Can you work these out from the model? Positions are in its coordinate system, mm. Face numbers are marked on the shaded views. A direction names the side the tool comes from. Coordinates: 2 decimals unless noted, no trailing zeros. Write each loop counter-clockwise with the first axis right and the second up, starting at its lowest first coordinate (ties: lowest second). Pieces come first, ordered by that corner, then holes. Notation, with made-up numbers: (-17, 86) -> (29, 86) arc R23 ccw to (29, 115) -> close; hole circle Ø11 at (73.25, -13.5). An arc over 180 degrees is marked (long way). Use one line per item in the form item = value.
```python
from build123d import *

# Parameters (mm, degrees)
SKETCH1_R           = 12
BOSS_EXTRUDE1_DEPTH = 5
BOSS_EXTRUDE2_DEPTH = 2
BOSS_EXTRUDE3_DEPTH = 2
SKETCH4_R           = 15.547757557
SKETCH4_R_2         = 12
BOSS_EXTRUDE4_DEPTH = 10
SKETCH5_W           = 10
SKETCH5_H           = 9.018962752
BOSS_EXTRUDE5_DEPTH = 2
SKETCH6_W           = 25.14370714
SKETCH6_H           = 10
BOSS_EXTRUDE6_DEPTH = 2
CUT_EXTRUDE1_DEPTH  = 2
CUT_EXTRUDE2_DEPTH  = 0.2


with BuildPart() as part:
    # Sketch1 → Boss-Extrude1 (new body)
    with BuildSketch(Plane.XY):
        with BuildLine():
            Line((-27.15, 21.666502105), (-25.112032094, 30.452193651))
            ThreePointArc((-25.112032094, 30.452193651), (-11.263369735, 42.043284959), (3.691801624, 31.919960581))
            Line((3.691801624, 31.919960581), (27.293258902, 23.278095711))
            Line((27.293258902, 23.278095711), (27.293258902, 10))
            Line((27.293258902, 10), (27.293258902, -9.955183239))
            Line((27.293258902, -9.955183239), (20.497693749, -9.955183239))
            Line((20.497693749, -9.955183239), (20.497693749, 10))
            Line((20.497693749, 10), (-20.5, 10))
            Line((-20.5, 10), (-20.5, -9.955183239))
            Line((-20.5, -9.955183239), (-27.15, -9.955183239))
            Line((-27.15, -9.955183239), (-27.15, 10))
            Line((-27.15, 10), (-27.15, 21.666502105))
        make_face()
        with Locations((-10.5, 27.062721997)):
            Circle(SKETCH1_R, mode=Mode.SUBTRACT)
    extrude(amount=BOSS_EXTRUDE1_DEPTH)

    # Sketch2 → Boss-Extrude2 (add)
    with BuildSketch(Plane(origin=(27.293258902, 0, 0), x_dir=(0, 0, -1), z_dir=(1, 0, 0))):
        Polygon((-5, -9.955183239), (-5, 23.278095711), (-15, 23.278095711), align=None)
    extrude(amount=-BOSS_EXTRUDE2_DEPTH)

    # Sketch3 → Boss-Extrude3 (add)
    with BuildSketch(Plane.ZY.offset(27.15)):
        Polygon((5, -9.955183239), (5, 23.278095711), (15, 23.278095711), align=None)
    extrude(amount=-BOSS_EXTRUDE3_DEPTH)

    # Sketch4 → Boss-Extrude4 (add)
    with BuildSketch(Plane.XY.offset(5)):
        with Locations((-10.5, 27.062721997)):
            Circle(SKETCH4_R)
        with Locations((-10.5, 27.062721997)):
            Circle(SKETCH4_R_2, mode=Mode.SUBTRACT)
    extrude(amount=BOSS_EXTRUDE4_DEPTH)

    # Sketch5 → Boss-Extrude5 (add)
    with BuildSketch(Plane(origin=(-30.532955865, 7.082559615, 0), x_dir=(0, 0, 1), z_dir=(-0.9741354729183627, 0.22596477690586622, 0))):
        with Locations((10, 21.050556457)):
            Rectangle(SKETCH5_W, SKETCH5_H)
    extrude(amount=-BOSS_EXTRUDE5_DEPTH)

    # Sketch6 → Boss-Extrude6 (add)
    with BuildSketch(Plane(origin=(10.742458336, 29.338305481, 0), x_dir=(0.9390305732894374, -0.34383365517021547, 0), z_dir=(0.34383365517021547, 0.9390305732894374, 0))):
        with Locations((5.053558251, -10)):
            Rectangle(SKETCH6_W, SKETCH6_H)
    extrude(amount=-BOSS_EXTRUDE6_DEPTH)

    # Sketch7 → Cut-Extrude1 (cut, along a direction that is not the sketch's normal)
    with BuildSketch(Plane(origin=(3.73770034, 16.113247996, 0), x_dir=(0.9741354729183627, -0.22596477690586628, -2.8423494966508805e-14), z_dir=(-0.2259647769058663, -0.9741354729183628, -1.225338527992233e-13))):
        Polygon((-29.99078277, 15), (-31.343644404, 15), (-31.343644404, 14.975239248), (-29.99078277, 14.883253417), align=None)
    extrude(amount=-CUT_EXTRUDE1_DEPTH, dir=(2.329279663418559e-14, -0.9575879123587351, -0.2881412676178814), mode=Mode.SUBTRACT)

    # Sketch8 → Cut-Extrude2 (cut)
    with BuildSketch(Plane.ZY.offset(25.477385016)):
        Polygon((15, 22.890108534), (15, 23.278095711), (14.883253417, 22.890108534), align=None)
    extrude(amount=-CUT_EXTRUDE2_DEPTH, mode=Mode.SUBTRACT)


solid = part.part
```
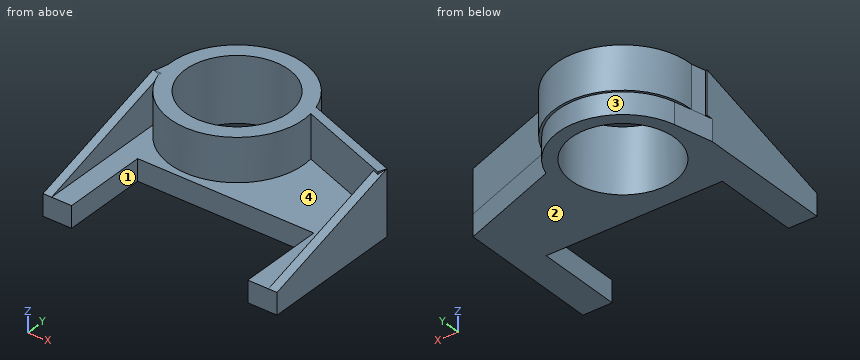
Q1. Suppose I cut it at B-B (y = 19). Write out the boundary of the cut face in (x, z).
Return value:
outline = (-27.15, 0) -> (-19.39, 0) -> (-19.39, 15) -> (-23.79, 15) -> (-23.79, 5) -> (-25.15, 5) -> (-25.15, 13.71) -> (-27.15, 13.71) -> close; (-1.61, 0) -> (27.29, 0) -> (27.29, 13.71) -> (25.29, 13.71) -> (25.29, 5) -> (2.79, 5) -> (2.79, 15) -> (-1.61, 15) -> close
Q2. Will these pins go through, and if not, where does the flat tip stop? pin 1 (4 mm diameter, centred on y = 32.5, z = 11, fed in from -X); pin 2 (5.5 mm diameter, centred on x = 8, z = 2.5, fed in from -Y); pin 3 (2 mm diameter, centred on x = -16.5, z = 8.5, fed in from +Y).
Return value:
pin_1 = -25.66
pin_2 = 10
pin_3 = 41.78
Q3. Suppose I cut it at A-A (x = -10.5). Write out the boundary of the cut face in (y, z).
Return value:
outline = (10, 0) -> (15.06, 0) -> (15.06, 15) -> (11.51, 15) -> (11.51, 5) -> (10, 5) -> close; (39.06, 0) -> (42.06, 0) -> (42.06, 5) -> (42.61, 5) -> (42.61, 15) -> (39.06, 15) -> close
Q4. For the marked faces 1, 2, 3 and 4, which set-ups out of +Z, -Z, +X, -X, +Y, -Y let a thin tool reach every point of the face, with its end or its side?
Return value:
face_1 = +Z, -Z, -Y
face_2 = -Z, +X, -X, +Y, -Y
face_3 = -Z, +Y
face_4 = +Z, -Y
Q5. Suppose I cut it at D-D (x = 0.5). Write out the boundary of the cut face in (y, z), then the cut area to 3 significant figures.
Return value:
outline = (10, 0) -> (22.27, 0) -> (22.27, 15) -> (16.07, 15) -> (16.07, 5) -> (10, 5) -> close; (31.86, 0) -> (37.26, 0) -> (37.26, 5) -> (38.05, 5) -> (38.05, 15) -> (31.86, 15) -> close
area = 212 mm2
Q6. If I drill on line 1 (Y direction, x = -10.5, z = 8.25); line 2 (X direction, y = 6, z = 5.5); line 3 (Y direction, x = -10.5, z = 4.25), over which ranges is the centre line in solid material (lowest first)? Write a range as from..to.
Return value:
line_1 = 11.51..15.06, 39.06..42.61
line_2 = -27.15..-25.15, 25.29..27.29
line_3 = 10..15.06, 39.06..42.06
Q7. Suppose I cut it at C-C (z = 8.5). Write out the boundary of the cut face in (x, y).
Return value:
outline = (-27.15, 1.68) -> (-25.15, 1.68) -> (-25.15, 21.86) arc R15.55 ccw to (4.88, 29.36) -> (25.29, 21.88) -> (25.29, 1.68) -> (27.29, 1.68) -> (27.29, 23.28) -> (4.35, 31.68) arc R15.55 ccw to (-26.04, 26.47) -> (-26.78, 23.28) -> (-27.15, 23.28) -> close; hole circle Ø24 at (-10.5, 27.06)
